Read the model definition and answer for the solid it produces. Units are mm, in the model's axes. Face numbers are marked on the shaded views. Coordinates: 2 decimals unless noted, no trailing zeros. Loops run counter-clockwise (first coordinate to the right, second up) from the corner with the lowest first, then second, coordinate; pieces in that order, holes last. Notation, with made-up numbers: (48, 7.5) -> (63, 7.5) arc R18 cw to (63, 33.5) -> close; hole circle Ø7 at (-12, 36.5). An arc over 180 degrees is marked (long way). Answer in a Markdown table with one row per item.
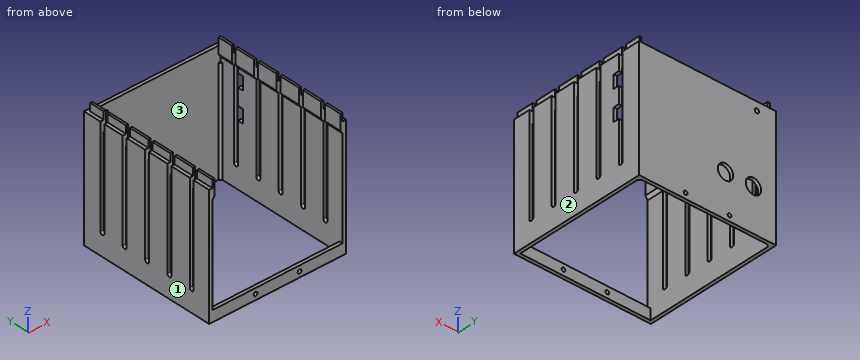
```python
from build123d import *

# Parameters (mm, degrees)
PAD_DEPTH           = 110
PAD001_DEPTH        = 96
SKETCH003_W         = 118.6
SKETCH003_H         = 10
PAD002_DEPTH        = 3
PAD003_DEPTH        = 123
POCKET001_DEPTH     = 124.601
LINEARPATTERN_COUNT = 5
LINEARPATTERN_PITCH = 22.5
SKETCH012_W         = 6
SKETCH012_H         = 12
POCKET_DEPTH        = 5
SKETCH013_R         = 1.7
POCKET004_DEPTH     = 126.001
SKETCH014_R         = 7
SKETCH014_R_2       = 2
POCKET005_DEPTH     = 5


with BuildPart() as part:
    # Sketch → Pad (new body)
    with BuildSketch(Plane.XY):
        Polygon((62.3, 64.5), (-62.3, 64.5), (-62.3, -61.5), (-59.3, -61.5), (-59.3, 61.5), (59.3, 61.5), (59.3, -61.5), (62.3, -61.5), align=None)
    extrude(amount=PAD_DEPTH)

    # Sketch001 → Pad001 (join)
    with BuildSketch(Plane.XY):
        Polygon((-59.3, 59.5), (-57.3, 61.5), (-59.3, 61.5), align=None)
    pad001 = extrude(amount=PAD001_DEPTH)

    # Mirrored: Pad001 across YZ
    add(pad001.mirror(Plane.YZ))

    # Sketch003 (on DatumPlane) → Pad002 (join)
    with BuildSketch(Plane.XZ.offset(61.5)):
        with Locations((0, 5)):
            Rectangle(SKETCH003_W, SKETCH003_H)
    extrude(amount=-PAD002_DEPTH)

    # Sketch004 (on DatumPlane) → Pad003 (join)
    with BuildSketch(Plane.XZ.offset(61.5)):
        Polygon((-57.3, 117), (-59.3, 117), (-59.3, 100), (-57.3, 103), align=None)
        Polygon((57.3, 103), (57.3, 117), (59.3, 117), (59.3, 100), align=None)
    extrude(amount=-PAD003_DEPTH)

    # Sketch009 (on DatumPlane) → Pocket001 (cut, through all)
    with BuildSketch(Plane.YZ.offset(62.3)):
        with BuildLine():
            Line((-46, 20), (-46, 243))
            ThreePointArc((-42, 243), (-44, 245), (-46, 243))
            Line((-42, 243), (-42, 20))
            ThreePointArc((-46, 20), (-44, 18), (-42, 20))
        make_face()
    pocket001 = extrude(amount=-POCKET001_DEPTH, mode=Mode.SUBTRACT)

    # LinearPattern: Pocket001 ×5
    with Locations(*[(0, i * LINEARPATTERN_PITCH, 0) for i in range(1, LINEARPATTERN_COUNT)]):
        add(pocket001, mode=Mode.SUBTRACT)

    # Sketch012 (on DatumPlane) → Pocket (cut)
    with BuildSketch(Plane.YZ.offset(62.3)):
        with Locations((41.830656, 89.723986)):
            Rectangle(SKETCH012_W, SKETCH012_H)
        with Locations((41.830656, 62.651357)):
            Rectangle(SKETCH012_W, SKETCH012_H)
    extrude(amount=-POCKET_DEPTH, mode=Mode.SUBTRACT)

    # Sketch013 (on DatumPlane) → Pocket004 (cut, through all)
    with BuildSketch(Plane.XZ.offset(-64.5)):
        with Locations((20, 5)):
            Circle(SKETCH013_R)
        with Locations((-20, 5)):
            Circle(SKETCH013_R)
    extrude(amount=POCKET004_DEPTH, mode=Mode.SUBTRACT)

    # Sketch014 (on DatumPlane) → Pocket005 (cut)
    with BuildSketch(Plane.XZ.offset(-64.5)):
        with Locations((-16.307726, 38.976202)):
            Circle(SKETCH014_R)
        with Locations((-41.748446, 38.976202)):
            Circle(SKETCH014_R)
        with Locations((-44.911871, 102.251883)):
            Circle(SKETCH014_R_2)
    extrude(amount=POCKET005_DEPTH, mode=Mode.SUBTRACT)


with BuildPart() as part_1:
    # Body placement: moved
    add(part.part.moved(Location((1.4, 0, 0))))


solid = part_1.part
```
1. Find the intervals of material crossed by probe 1 along X at (y, z) = (63.3, 5); probe 2 along X at (y, z) = (45, 6.5); probe 3 along Y at (x, z) = (-30, 5.5), in increasing order.
A:
| item | result |
|---|---|
| probe 1 | x = -60.9 to -20.3, -16.9 to 19.7, 23.1 to 63.7 |
| probe 2 | x = -60.9 to -57.9, 60.7 to 63.7 |
| probe 3 | y = -61.5 to -58.5, 61.5 to 64.5 |
2. The mould has two halves that part along X. Classify the marked faces 1, 2 and 3: pulls with the +X half, pulls with the -X half, needs draft (parallel to the pull), parting line crosses it, or undercut.
A:
| item | result |
|---|---|
| face 1 | pulls with the -X half |
| face 2 | pulls with the +X half |
| face 3 | undercut |
3. A cutting plane is placed at D-D on z = 5. Give the vertices of the cut face in (x, y), and give its area (3 significant figures).
A:
| item | result |
|---|---|
| outline | (-60.9, -61.5) -> (-20.3, -61.5) -> (-20.3, -58.5) -> (-57.9, -58.5) -> (-57.9, 59.5) -> (-55.9, 61.5) -> (-20.3, 61.5) -> (-20.3, 64.5) -> (-60.9, 64.5) -> close; (-16.9, -61.5) -> (19.7, -61.5) -> (19.7, -58.5) -> (-16.9, -58.5) -> close; (-16.9, 61.5) -> (19.7, 61.5) -> (19.7, 64.5) -> (-16.9, 64.5) -> close; (23.1, -61.5) -> (63.7, -61.5) -> (63.7, 64.5) -> (23.1, 64.5) -> (23.1, 61.5) -> (58.7, 61.5) -> (60.7, 59.5) -> (60.7, -58.5) -> (23.1, -58.5) -> close |
| area | 1,430 mm2 |
4. A cutting plane is placed at C-C on x = 4.5. Give the vertices of the cut face in (y, z).
A:
| item | result |
|---|---|
| outline | (-61.5, 0) -> (-58.5, 0) -> (-58.5, 10) -> (-61.5, 10) -> close; (61.5, 0) -> (64.5, 0) -> (64.5, 110) -> (61.5, 110) -> close |
5. A cutting plane is placed at B-B on x = 21.4. Give the vertices of the cut face in (y, z), and give its area (3 significant figures).
A:
| item | result |
|---|---|
| outline | (-61.5, 0) -> (-58.5, 0) -> (-58.5, 3.3) -> (-61.5, 3.3) -> close; (-61.5, 6.7) -> (-58.5, 6.7) -> (-58.5, 10) -> (-61.5, 10) -> close; (61.5, 0) -> (64.5, 0) -> (64.5, 3.3) -> (61.5, 3.3) -> close; (61.5, 6.7) -> (64.5, 6.7) -> (64.5, 110) -> (61.5, 110) -> close |
| area | 340 mm2 |
6. A cutting plane is placed at A-A on y = -32. Give the vertices of the cut face in (x, z), and give its area (3 significant figures).
A:
| item | result |
|---|---|
| outline | (-60.9, 0) -> (-57.9, 0) -> (-57.9, 100) -> (-55.9, 103) -> (-55.9, 117) -> (-57.9, 117) -> (-57.9, 110) -> (-60.9, 110) -> close; (58.7, 103) -> (60.7, 100) -> (60.7, 0) -> (63.7, 0) -> (63.7, 110) -> (60.7, 110) -> (60.7, 117) -> (58.7, 117) -> close |
| area | 722 mm2 |
7. Given pin 1 Ø18 at (x, z) = (-40.35, 38.98) entering from -Y; pin 2 Ø5.5 at (y, z) = (-8, 114.5) entering from -X; pin 3 Ø0.9 at (x, y) = (62.5, 9.5) entering from +Z, each flat-ended and moving along its own axis, determine where each tip first touches the part or whether it passes through.
A:
| item | result |
|---|---|
| pin 1 | stops at y = 61.5 |
| pin 2 | stops at x = -57.9 |
| pin 3 | stops at z = 110 |
